Autodesk Inventor part; units mm, degrees
ref_plane "YZ Plane" through (0, 0, 0) normal (1, 0, 0) x (0, 1, 0)
ref_plane "XZ Plane" through (0, 0, 0) normal (0, 1, 0) x (-1, 0, 0)
ref_plane "XY Plane" through (0, 0, 0) normal (0, 0, 1) x (1, 0, 0)
sketch "Sketch2" plane through (0, 0, 0) normal (1, 0, 0) x (0, 0, -1)
  line L0 (0, 0) -> (0, -18) construction
  line L1 (-8, 0) -> (-8, -18)
  line L2 (8, -18) -> (8, 0)
  arc A0 (8, 0) -> (-8, 0) centre (0, 0) ccw construction
  arc A1 (-8, -18) -> (8, -18) centre (0, -18) ccw construction
  arc A2 (5.5, -18) -> (-5.5, -18) centre (0, -18) ccw
  circle A3 centre (0, -18) radius 4.5 construction
  line L3 (-8, 0) -> (8, 0)
  line L4 (8, -18) -> (5.5, -18)
  arc A4 (-5.5, -18) -> (0, -23.5) centre (0, -18) ccw construction
  arc A5 (0, -23.5) -> (5.5, -18) centre (0, -18) ccw construction
  line L5 (-5.5, -18) -> (-8, -18)
  line L6 (5.5, -18) -> (-5.5, -18) construction
  line L7 (8, -18) -> (5.5, -18)
  line L8 (5.5, -18) -> (5.5, -22.5)
  line L9 (5.5, -22.5) -> (8, -22.5)
  line L10 (8, -22.5) -> (8, -18)
  line L11 (-8, -18) -> (-5.5, -18)
  line L12 (-5.5, -18) -> (-5.5, -22.5)
  line L13 (-5.5, -22.5) -> (-8, -22.5)
  line L14 (-8, -22.5) -> (-8, -18)
  point P0 (0, -9)
  dimension "d2" = 2.5
  dimension "d3" = 9
  dimension "d4" = 1
  dimension "d5" = 18
  dimension "d18" = 4.5
extrude "Extrusion1" add sketch "Sketch2" along normal mid plane 8
sketch "Sketch3" plane through (4, 0, 8) normal (0, 1, 0) x (0, 0, -1)
  line L0 (-7, 0) -> (23, 0)
  line L1 (23, 0) -> (23, 8)
  line L2 (23, 8) -> (-7, 8)
  line L3 (-7, 8) -> (-7, 0)
  line L4 (-7, 0) -> (23, 8) construction
  line L5 (23, 0) -> (-7, 8) construction
  line L6 (0, 8) -> (16, 8)
  line L7 (0, 8) -> (0, 0)
  point P0 (8, 4)
  dimension "d8" = 7
extrude "Extrusion2" add sketch "Sketch3" against normal blind 2
sketch "Sketch4" plane through (4, -2, 8) normal (0, -1, 0) x (0, 0, -1)
  line L0 (23, 0) -> (23, -8)
  line L1 (23, -8) -> (16, -8)
  line L2 (16, -8) -> (0, -8)
  line L3 (0, -8) -> (0, 0)
  line L4 (-7, 0) -> (0, 0)
  line L5 (-7, -8) -> (-7, 0)
  line L6 (0, -8) -> (-7, -8)
  line L7 (16, 0) -> (23, 0)
  line L8 (16, 0) -> (16, -8)
  line L9 (0, 0) -> (16, 0)
  point P0 (19.5, -4)
  point P1 (19.5, -8)
  point P2 (23, -4)
  point P3 (-3.5, -4)
  point P4 (-7, -4)
  point P5 (-3.5, -8)
hole "Hole1" at (0, -2, -11.5) at (0, -2, 11.5) direction (0, 1, 0) diameter 3.4 end through all
chamfer "Chamfer1" distance 1 angle 45 2 edges at (0, -22.5, -8) (0, -22.5, 8)
equation "\"d18\" = 0.5 * d3"
properties part number "differential stopper"
Here's how the part is built. I have some questions about the finished solid (model axes, mm). A direction names the side the tool comes from. Coordinates: 2 decimals unless noted, no trailing zeros. Loops run counter-clockwise (first coordinate to the right, second up) from the corner with the lowest first, then second, coordinate; pieces in that order, holes last. Notation, with made-up numbers: (-21, 43.5) -> (4, 43.5) arc R25 cw to (4, 79.5) -> close; hole circle Ø3 at (-13, -12.75). An arc over 180 degrees is marked (long way). Use one line per item in the form item = value. Start each with the question number.
(1) If we section it at B-B (x = 0): Please give me the cut outline in (y, z), then the cut area to 3 significant figures.
(2) If we section it at C-C (x = -2.25): Please give me the cut outline in (y, z), then the cut area to 3 significant figures.
(3) If we section it at D-D (y = -16): Please give me the cut outline in (x, z), then the cut area to 3 significant figures.
(4) Will these pins go through, and if not, where does the flat tip stop? pin 1 (1 mm diameter, centred on x = -2, z = -4, fed in from -Y); pin 2 (2.5 mm diameter, centred on x = -0.5, y = -8.5, fed in from +Z); pin 3 (1 mm diameter, centred on x = -3, y = -3, fed in from -Z).
(5) If we section it at A-A (z = 11.5): Please give me the cut outline in (x, y), then the cut area to 3 significant figures.
(6) Please list where these lines run through material, in increasing order: line 1 along Z through (x, y) = (0, -0.7); line 2 along X through (y, z) = (-1.5, 11.5); line 3 along Y through (x, z) = (1, 13.5).
(7) On a 3-axis mill with a long thin cutter (end or side, diameter ignored), from which of +Z, -Z, +X, -X, +Y, -Y can I reach the whole of each face in a straight line? I mean faces 5 (the face through (0.65, -0.99, -13.07)), 6 (the face through (0, -20, 5.5)), 7 (the face through (-2, -2, -11)), 8 (the face through (0, 0, 0)), 9 (the face through (0, -12, 8)). Say none if no direction works.
(8) We'd pull the mould along X, two halves only. Please class faces 1 (the face through (-4, -9, 0)), 2 (the face through (-0.51, -0.99, 9.88)), 3 (the face through (4, -9, 0)), 4 (the face through (0, -1, -15)): pulls with the +X half, pulls with the -X half, needs draft (parallel to the pull), parting line crosses it, or undercut.
Verdict:
q1.outline = (-22.5, -7) -> (-21.5, -8) -> (-2, -8) -> (-2, -9.8) -> (0, -9.8) -> (0, 9.8) -> (-2, 9.8) -> (-2, 8) -> (-21.5, 8) -> (-22.5, 7) -> (-22.5, 5.5) -> (-18, 5.5) arc R5.5 cw to (-18, -5.5) -> (-22.5, -5.5) -> close; (-2, -15) -> (0, -15) -> (0, -13.2) -> (-2, -13.2) -> close; (-2, 13.2) -> (0, 13.2) -> (0, 15) -> (-2, 15) -> close
q1.area = 276 mm²
q2.outline = (-22.5, -7) -> (-21.5, -8) -> (-2, -8) -> (-2, -15) -> (0, -15) -> (0, 15) -> (-2, 15) -> (-2, 8) -> (-21.5, 8) -> (-22.5, 7) -> (-22.5, 5.5) -> (-18, 5.5) arc R5.5 cw to (-18, -5.5) -> (-22.5, -5.5) -> close
q2.area = 290 mm²
q3.outline = (-4, -8) -> (4, -8) -> (4, -5.12) -> (-4, -5.12) -> close; (-4, 5.12) -> (4, 5.12) -> (4, 8) -> (-4, 8) -> close
q3.area = 46.0 mm²
q4.pin_1 = -14.84
q4.pin_2 = 8
q4.pin_3 = -8
q5.outline = (-4, -2) -> (-1.7, -2) -> (-1.7, 0) -> (-4, 0) -> close; (1.7, -2) -> (4, -2) -> (4, 0) -> (1.7, 0) -> close
q5.area = 9.20 mm²
q6.line_1 = -15 to -13.2, -9.8 to 9.8, 13.2 to 15
q6.line_2 = -4 to -1.7, 1.7 to 4
q6.line_3 = -2 to 0
q7.face_5 = +Y, -Y
q7.face_6 = +X, -X, -Y
q7.face_7 = -Z, +X, -X, -Y
q7.face_8 = +Z, -Z, +X, -X, +Y
q7.face_9 = +Z, +X, -X, -Y
q8.face_1 = pulls with the -X half
q8.face_2 = undercut
q8.face_3 = pulls with the +X half
q8.face_4 = needs draft
